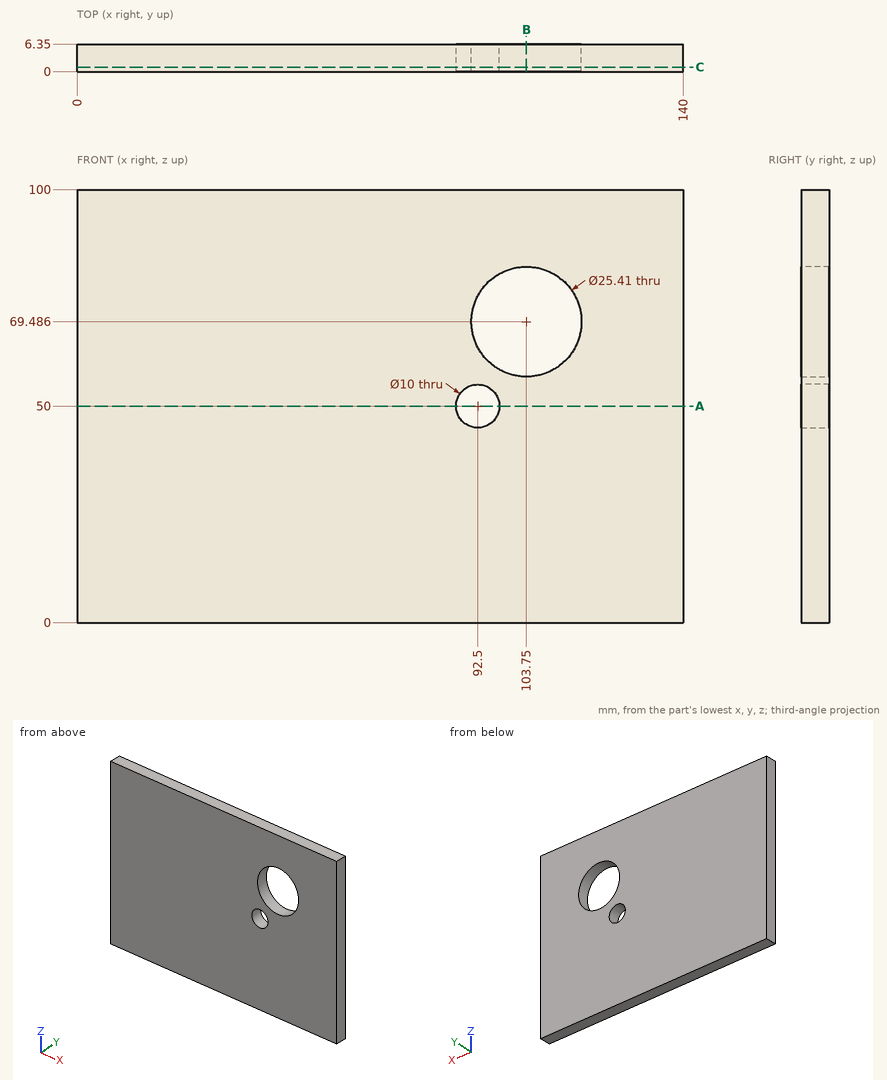
For this review, use the dimensioned drawing (mm, ordinates from the lowest corner) and the shaded views. Coordinates: 2 decimals unless noted, no trailing zeros. Order: outer loops, then holes, each group sorted by start corner. A loop starts at its lowest first (then second) coordinate and runs counter-clockwise, first axis right, second up. Notation, with made-up numbers: (86.25, 73) - (112.25, 73) arc R16 ccw to (112.25, 91) - close; hole circle Ø5 at (-37.75, 68). An arc over 180 degrees is marked (long way). Answer as a JSON object with one key per item and string values. Group by question number.
1. For probe 1 along X at (y, z) = (2, 50); probe 2 along Z at (x, y) = (96, 2.25) (1 decimal); probe 3 along X at (y, z) = (2.5, 76), list the stretches that pass through material, from the lowest coordinate up.
2. We need section A-A on z = 50. State the section outline as (x, y) points.
3. We need section C-C on y = 1. Give the number of separate pieces and of enclosed holes in the cut face, then the cut area to 3 significant figures.
4. We need section B-B on x = 103.75. State the section outline as (y, z) points.
Final values:
{
 "1": {"probe 1": "0 to 87.5, 97.5 to 140", "probe 2": "0 to 46.4, 53.6 to 59.4, 79.6 to 100", "probe 3": "0 to 92.84, 114.66 to 140"},
 "2": {"outline": "(0, 0) - (87.5, 0) - (87.5, 6.35) - (0, 6.35) - close; (97.5, 0) - (140, 0) - (140, 6.35) - (97.5, 6.35) - close"},
 "3": {"separate pieces": "1", "enclosed holes": "2", "area": "13,400 mm²"},
 "4": {"outline": "(0, 0) - (6.35, 0) - (6.35, 56.78) - (0, 56.78) - close; (0, 82.19) - (6.35, 82.19) - (6.35, 100) - (0, 100) - close"}
}
